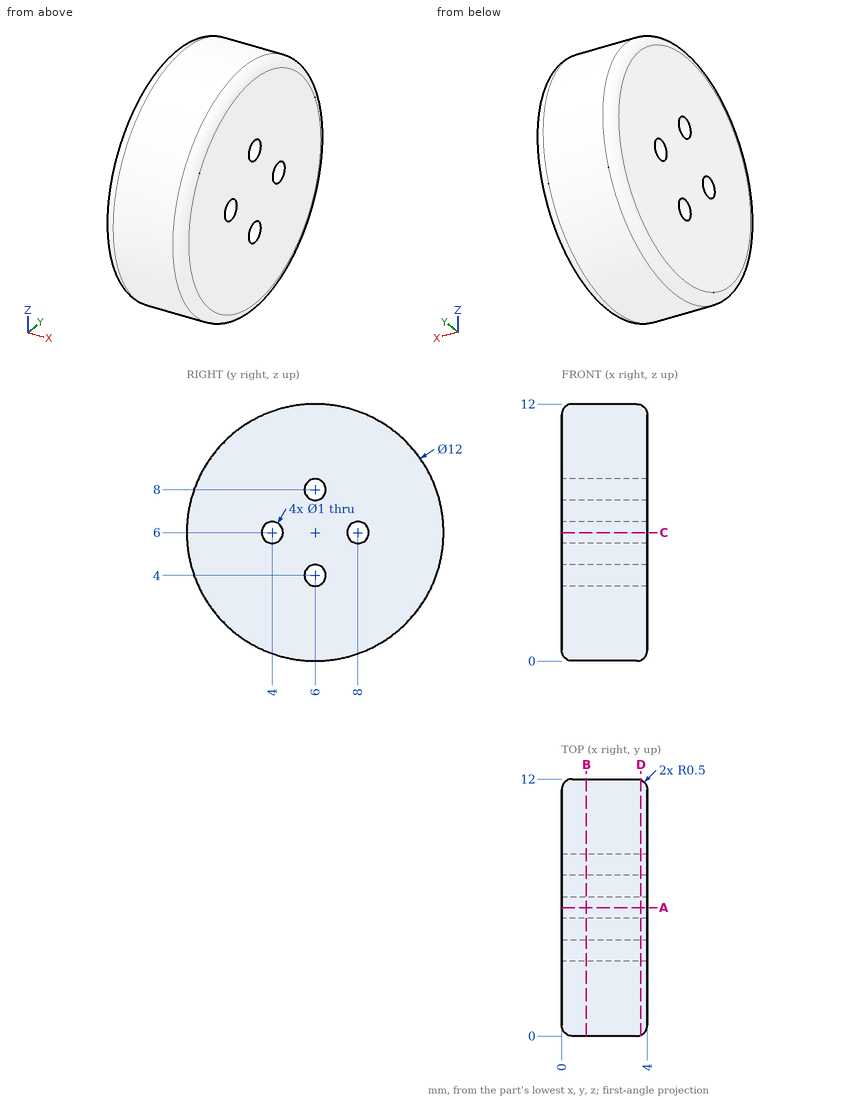
Design review of the part shown in the three views and the two pictorial views. Dimensions are in mm from the part's minimum x, y and z. Round coordinates to 2 decimals unless told otherwise and drop trailing zeros. Loops run counter-clockwise (first coordinate to the right, second up) from the corner with the lowest first, then second, coordinate; pieces in that order, holes last. Notation, with made-up numbers: (9, -3) - (19, -3) arc R29 ccw to (19, 28) - close; hole circle Ø11 at (-2.5, 56). An arc over 180 degrees is marked (long way). Answer as CSV lines item,"result".
(1) Consider section B-B on x = 1.15. Give the boundary of the cut face in (y, z), then the cut area to 3 significant figures.
Checked values:
outline,"circle Ø12 at (6, 6); hole circle Ø1 at (4, 6); hole circle Ø1 at (6, 4); hole circle Ø1 at (6, 8); hole circle Ø1 at (8, 6)"
area,"110 mm2"
(2) Consider section D-D on x = 3.7. Give the boundary of the cut face in (y, z).
Checked values:
outline,"circle Ø11.92 at (6, 6); hole circle Ø1 at (4, 6); hole circle Ø1 at (6, 4); hole circle Ø1 at (6, 8); hole circle Ø1 at (8, 6)"
(3) Consider section C-C on z = 6. Give the number of separate pieces and of enclosed holes in the cut face, then the cut area to 3 significant figures.
Checked values:
separate pieces,"3"
enclosed holes,"0"
area,"39.8 mm2"
(4) Wall thickness on line 1 (Z direction, x = 2.95, y = 6); line 2 (Z direction, x = 3.8, y = 3.75); line 3 (Z direction, x = 0.25, y = 8): over which ranges is each line inside the solid? List them lowest first.
Checked values:
line 1,"z = 0 to 3.5, 4.5 to 7.5, 8.5 to 12"
line 2,"z = 0.55 to 5.57, 6.43 to 11.45"
line 3,"z = 0.41 to 5.5, 6.5 to 11.59"
(5) Consider section A-A on y = 6. Give the boundary of the cut face in (x, z), then the cut area to 3 significant figures.
Checked values:
outline,"(0, 0.5) arc R0.5 ccw to (0.5, 0) - (3.5, 0) arc R0.5 ccw to (4, 0.5) - (4, 3.5) - (0, 3.5) - close; (0, 4.5) - (4, 4.5) - (4, 7.5) - (0, 7.5) - close; (0, 8.5) - (4, 8.5) - (4, 11.5) arc R0.5 ccw to (3.5, 12) - (0.5, 12) arc R0.5 ccw to (0, 11.5) - close"
area,"39.8 mm2"
(6) Insertion check: P1, Ø1.5, axis at x = 1, z = 2, coming from the +Y side; P2, Ø1.5, axis at y = 7, z = 1.5, coming from the -X side. Each pin has a flat end and moves straight along its axis. Give the tip position at first contact, or say it passes through.
Checked values:
P1,"stops at y = 11.04"
P2,"stops at x = 0"
